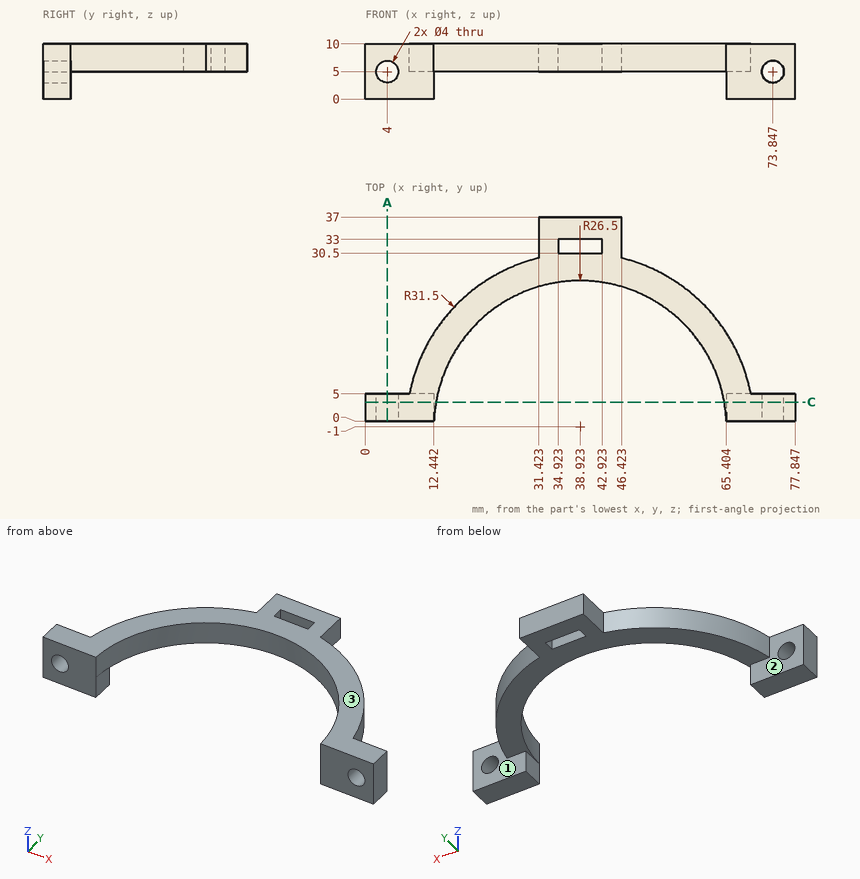
Check sheet for the drawn part. Datum: minimum x, y, z corner. Units: mm. A direction names the side the tool comes from. Give positions to 0.01 mm unless a question says otherwise; leave off trailing zeros. Order: outer loops, then holes, each group sorted by start corner. A loop starts at its lowest first (then second) coordinate and runs counter-clockwise, first axis right, second up. Notation, with made-up numbers: (82.25, -37.75) - (122.25, -37.75) arc R11 ccw to (122.25, -16.75) - close; hole circle Ø8 at (64.25, 7.25). An arc over 180 degrees is marked (long way). Answer as a JSON object with one key per item and string values.
(1) Tool access check on the marked faces 1, 2 and 3. Record the directions out of +Z, -Z, +X, -X, +Y, -Y that give a thin tool (end or side, any length) a straight path to the whole face; none if there is none.
Report:
{"face 1": "-Z, +X, +Y", "face 2": "-Z, -X, +Y", "face 3": "+Z, +X, -X, +Y, -Y"}
(2) Material ranges on line 1 (Z direction, x = 4, y = 3.7); line 2 (Y direction, x = 3, z = 9.5); line 3 (X direction, y = 11.5, z = 6) (1 decimal), recorded low to high.
Report:
{"line 1": "0 to 3, 7 to 10", "line 2": "0 to 5", "line 3": "10 to 15.6, 62.3 to 67.8"}
(3) Cross-section at C-C (y = 3.5). State how many separate pieces and enclosed holes the cut face has, then the cut area to 3 significant figures.
Report:
{"separate pieces": "2", "enclosed holes": "2", "area": "227 mm^2"}
(4) Cross-section at A-A (x = 4). Record the cut outline in (y, z), then the cut area to 3 significant figures.
Report:
{"outline": "(0, 0) - (5, 0) - (5, 3) - (0, 3) - close; (0, 7) - (5, 7) - (5, 10) - (0, 10) - close", "area": "30.0 mm^2"}
(5) Depth check by flat-ended pin: pin 1 Ø5 at (y, z) = (27, 4) entering from +X (1 decimal); pin 2 Ø8 at (x, y) = (35, 20.5) entering from +Z; pin 3 Ø3 at (y, z) = (32, 7.5) entering from -X; pin 4 Ø2.5 at (y, z) = (2, 3) entering from -X. Enter the tip coordinate at first touch or a pass-through.
Report:
{"pin 1": "x = 57.1", "pin 2": "through", "pin 3": "x = 31.42", "pin 4": "x = 0"}
